Source: CAD feature listing. Evaluate the final solid. Frame: model axes, mm. A direction names the side the tool comes from. Coordinates: 2 decimals unless noted, no trailing zeros. Order: outer loops, then holes, each group sorted by start corner. A loop starts at its lowest first (then second) coordinate and runs counter-clockwise, first axis right, second up. Notation, with made-up numbers: (-10.5, 56.25) - (18.5, 56.25) arc R32 cw to (18.5, 87.25) - close; hole circle Ø9 at (-31, 74). An arc over 180 degrees is marked (long way). One line per question, with ' | ' between items. Start each with the question number.
(1) Section A-A (x = -23.5). Return the cut outline in (y, z), then the cut area to 3 significant figures.
(2) Line query: line 1 along Y through (x, z) = (-4.2, 13.4); line 2 along Z through (x, y) = (-4, -3); line 3 along Z through (x, y) = (-1.55, -3.6). Output: solid intervals per line, ascending.
(3) Contact query for flat-ended pins moving along their axis: P1, Ø20, axis at x = -15.5, y = -10, coming from the +Z side; P2, Ø1.8, axis at y = -15, z = 0.5, coming from the +X side; P3, Ø10, axis at y = -7.5, z = 18, coming from the -X side. Output: stop coordinate, or through.
(4) Section C-C (y = -3.6). Return the cut outline in (x, z).
(5) Section D-D (z = 4). Return the cut outline in (x, y).
(6) Draft query along X for faces 1 (the flat face through (-3.2, -13, 21)), 2 (the flat face through (2, -16.8, 4.1)), 3 (the cylindrical face through (-22.828, -15.946, 0.789)), 4 (the flat face through (-2, -17, 19.9)). Return one class per face: +X half, -X half, draft (parallel to the pull), parting line (faces both ways), or undercut.
(7) Access query for faces 5 (the flat face through (9.8, -26.55, 0.79)), 6 (the flat face through (9, -3, 1.6)), 7 (the flat face through (-5.2, -4, 12)). Directions: +Z, -Z, +X, -X, +Y, -Y. A direction counts if a zero-diameter tool reaches every point of the face in a straight line with its end or side. Return the directions, or none.
(8) Section B-B (y = -23.5). Return the cut outline in (x, z).
from build123d import *

# Parameters (mm, degrees)
PAD_DEPTH       = 34
SKETCH_R        = 0.9
POCKET_DEPTH    = 22.001
SKETCH003_W     = 13
SKETCH003_H     = 23.2
POCKET001_DEPTH = 22.001
SKETCH005_R     = 1.25
PAD001_DEPTH    = 1.6
SKETCH006_R     = 1.25
PAD002_DEPTH    = 1.6
SKETCH008_R     = 1.8
SKETCH008_R_2   = 1
PAD003_DEPTH    = 2
CHAMFER_SIZE    = 3
CHAMFER001_SIZE = 12


with BuildPart() as part:
    # Sketch001 → Pad (new body)
    with BuildSketch(Plane.XZ):
        Polygon((-22, 1.6), (-8.2, 1.6), (-3.2, 6.6), (-3.2, 22.2), (0, 22.2), (0, 6.6), (4, 1.6), (4, 0), (-3.601763, 0), (-22, 0), align=None)
    extrude(amount=PAD_DEPTH)

    # Sketch → Pocket (cut, through all)
    with BuildSketch(Plane(origin=(0, 0, 0), x_dir=(0, 0, 1), z_dir=(1, 0, 0))):
        with Locations((13.4, 30.8)):
            Circle(SKETCH_R)
        with Locations((13.4, 3.6)):
            Circle(SKETCH_R)
    extrude(amount=-POCKET_DEPTH, mode=Mode.SUBTRACT)

    # Sketch003 (on DatumPlane) → Pocket001 (cut, through all)
    with BuildSketch(Plane(origin=(0, 0, 0), x_dir=(0, 0, 1), z_dir=(1, 0, 0))):
        with Locations((13.4, 17.2)):
            Rectangle(SKETCH003_W, SKETCH003_H)
    extrude(amount=-POCKET001_DEPTH, mode=Mode.SUBTRACT)

    # Sketch005 → Pad001 (join)
    with BuildSketch(Plane.XY):
        with BuildLine():
            ThreePointArc((-24.911765, -14.352941), (-26.5, -17), (-24.911765, -19.647059))
            Line((-20.5, -22), (-24.911765, -19.647059))
            Line((-20.5, -12), (-20.5, -22))
            Line((-20.5, -12), (-24.911765, -14.352941))
        make_face()
        with Locations((-23.5, -17)):
            Circle(SKETCH005_R, mode=Mode.SUBTRACT)
    extrude(amount=PAD001_DEPTH)

    # Sketch006 → Pad002 (join)
    with BuildSketch(Plane.XY):
        with BuildLine():
            ThreePointArc((15, -34), (17.975766, -31.380547), (15.754946, -28.096544))
            Line((0, -24), (15.754946, -28.096544))
            Line((0, -34), (0, -24))
            Line((0, -34), (15, -34))
        make_face()
        with Locations((15, -31)):
            Circle(SKETCH006_R, mode=Mode.SUBTRACT)
        with BuildLine():
            ThreePointArc((15.754946, -5.903456), (17.975766, -2.619453), (15, 0))
            Line((0, 0), (15, 0))
            Line((0, 0), (0, -10))
            Line((0, -10), (15.754946, -5.903456))
        make_face()
        with Locations((15, -3)):
            Circle(SKETCH006_R, mode=Mode.SUBTRACT)
    extrude(amount=PAD002_DEPTH)

    # Sketch008 (on Face2 of Pad002) → Pad003 (join)
    with BuildSketch(Plane(origin=(-3.2, 0, 0), x_dir=(0, 0, -1), z_dir=(-1, 0, 0))):
        with Locations((-13.4, 30.8)):
            Circle(SKETCH008_R)
        with Locations((-13.4, 30.8)):
            Circle(SKETCH008_R_2, mode=Mode.SUBTRACT)
        with Locations((-13.4, 3.6)):
            Circle(SKETCH008_R)
        with Locations((-13.4, 3.6)):
            Circle(SKETCH008_R_2, mode=Mode.SUBTRACT)
    extrude(amount=PAD003_DEPTH)

    # Chamfer
    chamfer_edges = [part.edges().sort_by_distance(p)[0] for p in [
        (-1.6, -34, 22.2),
        (-1.6, 0, 22.2),
    ]]
    chamfer(chamfer_edges, length=CHAMFER_SIZE)

    # Chamfer001
    chamfer001_edges = [part.edges().sort_by_distance(p)[0] for p in [
        (-22, -34, 0.8),
        (-22, 0, 0.8),
    ]]
    chamfer(chamfer001_edges, length=CHAMFER001_SIZE)


solid = part.part
Response values:
1) outline: (-20.4, 0) - (-18.25, 0) - (-18.25, 1.6) - (-20.4, 1.6) - close; (-15.75, 0) - (-13.6, 0) - (-13.6, 1.6) - (-15.75, 1.6) - close | area: 6.88 mm²
2) line 1: y = -32.6 to -31.8, -29.8 to -29, -5.4 to -4.6, -2.6 to -1.8 | line 2: z = 0 to 5.8, 11.7 to 12.6, 14.2 to 15.1 | line 3: z = 0 to 12.5, 14.3 to 22.2
3) P1: stops at z = 4.3 | P2: stops at x = 4 | P3: stops at x = -5.2
4) outline: (-13.6, 0) - (13.9, 0) - (13.9, 1.6) - (4, 1.6) - (0, 6.6) - (0, 12.5) - (-3.2, 12.5) - (-3.2, 12.4) - (-5.2, 12.4) - (-5.2, 11.6) - (-3.2, 11.6) - (-3.2, 6.6) - (-8.2, 1.6) - (-13.6, 1.6) - close; (-5.2, 14.4) - (-3.2, 14.4) - (-3.2, 14.3) - (0, 14.3) - (0, 22.2) - (-3.2, 22.2) - (-3.2, 15.2) - (-5.2, 15.2) - close; (16.1, 0) - (17.94, 0) - (17.94, 1.6) - (16.1, 1.6) - close
5) outline: (-5.8, -34) - (2.08, -34) - (2.08, 0) - (-5.8, 0) - close
6) face 1: -X half | face 2: +X half | face 3: undercut | face 4: draft
7) face 5: +Z, -Z, +X | face 6: +Z, +X, +Y, -Y | face 7: +Z, -X, +Y, -Y
8) outline: (-20.5, 0) - (4, 0) - (4, 1.6) - (0, 6.6) - (0, 6.9) - (-3.2, 6.9) - (-3.2, 6.6) - (-8.2, 1.6) - (-20.5, 1.6) - close; (-3.2, 19.9) - (0, 19.9) - (0, 22.2) - (-3.2, 22.2) - close
